Here's the drawing with two shaded views (mm, measured from the low corner). I have some questions. Round coordinates to 2 decimals unless told otherwise and drop trailing zeros. Order: outer loops, then holes, each group sorted by start corner. A loop starts at its lowest first (then second) coordinate and runs counter-clockwise, first axis right, second up. Notation, with made-up numbers: (42.5, 76.25) -> (47.5, 76.25) arc R30 cw to (47.5, 110.25) -> close; hole circle Ø2 at (71, 43). An arc over 180 degrees is marked (long way). Use a Markdown table: item, result. Add a question column.
Q1. I'm going to push a flat-ended pin straight in: pin 1 Ø2.5 at (x, z) = (7.5, 30) entering from +Y (1 decimal). Where does the tip first touch, or does it pass through?
Q2. If we section it at A-A on z = 8: List the corners of the cut face in (x, y) for me, plus the area to 3 significant figures.
Q3. If we section it at B-B on x = 7.5: List the corners of the cut face in (y, z) for me, plus the area to 3 significant figures.
Q4. If we section it at C-C on y = 0.8: List the corners of the cut face in (x, z) for me, plus the area to 3 significant figures.
Q5. If we section it at D-D on z = 30: List the corners of the cut face in (x, y) for me, plus the area to 3 significant figures.
Q6. I need wall thicknesses on line 1 along Z through (x, y) = (7.5, 1.2); line 2 along X through (y, z) = (1.05, 30); line 3 along X through (y, z) = (1.2, 8). Which ranges of each line are inside material? Lowest first, please. Write a range as [from, to].
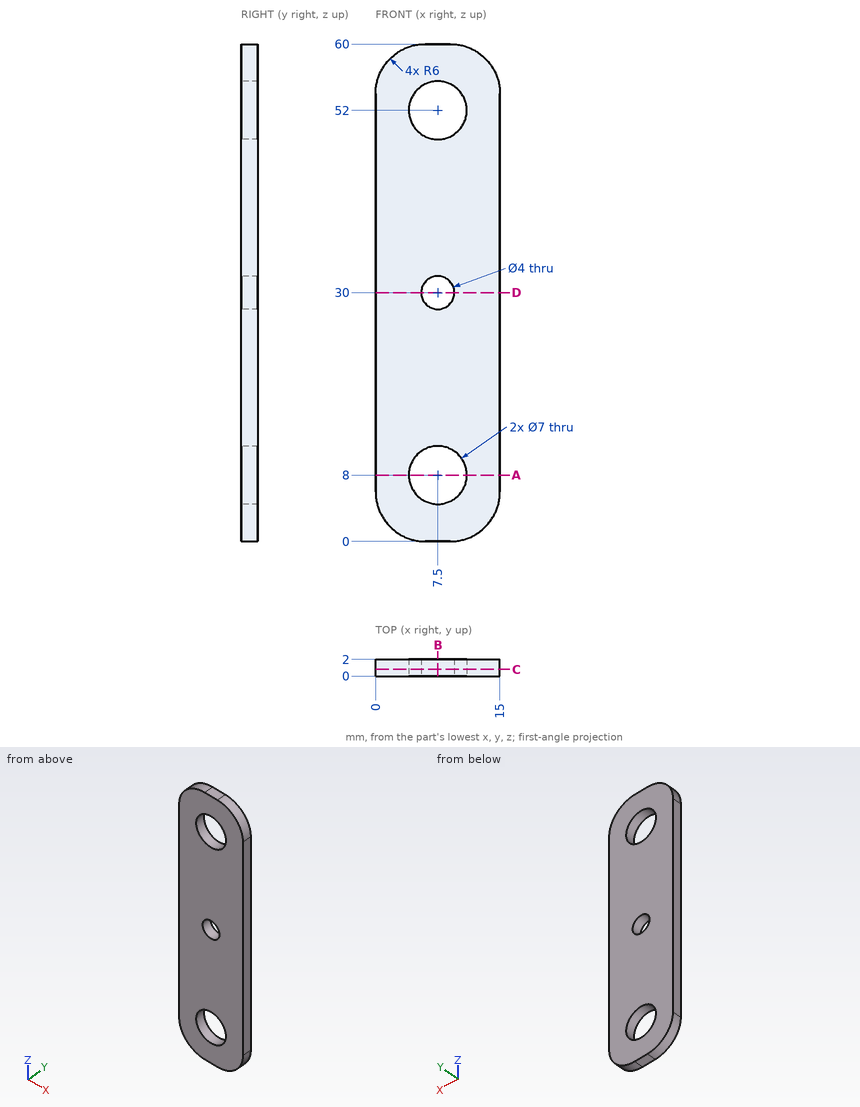
Answer below:
| question | item | result |
|---|---|---|
| 1 | pin 1 | through |
| 2 | outline | (0, 0) -> (4, 0) -> (4, 2) -> (0, 2) -> close; (11, 0) -> (15, 0) -> (15, 2) -> (11, 2) -> close |
| 2 | area | 16.0 mm² |
| 3 | outline | (0, 0) -> (2, 0) -> (2, 4.5) -> (0, 4.5) -> close; (0, 11.5) -> (2, 11.5) -> (2, 28) -> (0, 28) -> close; (0, 32) -> (2, 32) -> (2, 48.5) -> (0, 48.5) -> close; (0, 55.5) -> (2, 55.5) -> (2, 60) -> (0, 60) -> close |
| 3 | area | 84.0 mm² |
| 4 | outline | (0, 6) arc R6 ccw to (6, 0) -> (9, 0) arc R6 ccw to (15, 6) -> (15, 54) arc R6 ccw to (9, 60) -> (6, 60) arc R6 ccw to (0, 54) -> close; hole circle Ø7 at (7.5, 8); hole circle Ø7 at (7.5, 52); hole circle Ø4 at (7.5, 30) |
| 4 | area | 780 mm² |
| 5 | outline | (0, 0) -> (5.5, 0) -> (5.5, 2) -> (0, 2) -> close; (9.5, 0) -> (15, 0) -> (15, 2) -> (9.5, 2) -> close |
| 5 | area | 22.0 mm² |
| 6 | line 1 | [0, 4.5], [11.5, 28], [32, 48.5], [55.5, 60] |
| 6 | line 2 | [0, 5.5], [9.5, 15] |
| 6 | line 3 | [0, 4], [11, 15] |
